The listing builds one solid part. Answer for the finished solid, in the listing's coordinates (mm). A direction names the side the tool comes from. Give positions to 0.01 mm unless a question says otherwise; leave off trailing zeros. Loops run counter-clockwise (first coordinate to the right, second up) from the corner with the lowest first, then second, coordinate; pieces in that order, holes last.
Item 1: Section B-B, the plane y = 0 is taken. Give the vertices of the cut face in (x, z).
Item 2: A tool of negligible diameter and unlimited length cuts with its end or side. For faces 1 (the face through (-5, -1, 8)), 2 (the face through (-2.1, 1.3, 6.7)), 3 (the face through (-1.287, 0.103, 5.179)), 4 (the face through (-5, 1, 8)), 5 (the face through (-7, 0, 9.7)), from which of +Z, -Z, +X, -X, +Y, -Y can it reach the whole face along a straight path? Write none if from no direction.
Item 3: Consider line 1 along X through (y, z) = (0, 6); line 2 along Z through (x, y) = (-2.25, 1.5); line 3 along X through (y, z) = (0, 7.5). Determine where each line is inside the solid, lowest interval first.
Item 4: Section A-A, the plane z = 6.25 is taken. Give the vertices of the cut face in (x, y), and give its area (3 significant figures).
Item 5: Section C-C, the plane x = 1.5 is taken. Give the vertices of the cut face in (y, z).
Item 6: Section D-D, the plane z = 7.25 is taken. Give the vertices of the cut face in (x, y), and give its area (3 significant figures).
Item 7: The mould has two halves that part along Y. Classify faces 6 (the face through (-6.171, 2.177, 4.317)), 7 (the face through (-4, 0, 2)), 8 (the face through (1, -2, 3.5)): pulls with the +Y half, pulls with the -Y half, needs draft (parallel to the pull), parting line crosses it, or undercut.
Item 8: Each of these flat-tipped pins is pushed along its axis until it touches: pin 1 Ø1.4 at (x, y) = (0, -0.5) entering from +Z; pin 2 Ø4 at (y, z) = (2, 7) entering from -X; pin 3 Ø2.5 at (x, y) = (1.06, 0) entering from +Z; pin 4 Ø1.5 at (x, z) = (-4, 8) entering from -Y. Where does it stop, or does it pass through?
from build123d import *
from build123d.topology import SkipClean

# Parameters (mm, degrees)
SKETCH1_R           = 2.35
BOSS_EXTRUDE1_DEPTH = 6.7
BOSS_EXTRUDE2_DEPTH = 3
CUT_EXTRUDE1_DEPTH  = 2
SKETCH4_R           = 2.35
SKETCH4_R_2         = 1.45
BOSS_EXTRUDE3_DEPTH = 1.5


with BuildPart() as part:
    # Sketch1 → Boss-Extrude1 (new body)
    with BuildSketch(Plane.XY):
        with BuildLine():
            Line((-1.533260445, 2.35), (-10.939517975, 2))
            ThreePointArc((-10.939517975, 2), (-12.939517975, 0), (-10.939517975, -2))
            Line((-10.939517975, -2), (-1.533260445, -2.35))
            ThreePointArc((-1.533260445, -2.35), (4.560482025, 0), (-1.533260445, 2.35))
        make_face()
        with Locations((1.060482025, 0)):
            Circle(SKETCH1_R, mode=Mode.SUBTRACT)
    extrude(amount=BOSS_EXTRUDE1_DEPTH)

    # Sketch2 → Boss-Extrude2 (add)
    with SkipClean():  # the faces are left unmerged after this step: merging them gives an invalid solid
        with BuildSketch(Plane.XY.offset(6.7)):
            with BuildLine():
                Line((-8.939517975, 1), (-1.289517975, 1))
                ThreePointArc((-1.289517975, 1), (-1.18252076, 0.99425932), (-1.076752018, 0.977103192))
                ThreePointArc((-1.076752018, 0.977103192), (-1.289517975, 0), (-1.076752018, -0.977103192))
                ThreePointArc((-1.076752018, -0.977103192), (-1.18252076, -0.99425932), (-1.289517975, -1))
                Line((-1.289517975, -1), (-8.939517975, -1))
                ThreePointArc((-8.939517975, -1), (-9.065522268, -0.992029696), (-9.189517975, -0.968245837))
                ThreePointArc((-9.189517975, -0.968245837), (-12.939517975, 0), (-9.189517975, 0.968245837))
                ThreePointArc((-9.189517975, 0.968245837), (-9.065522268, 0.992029696), (-8.939517975, 1))
            make_face()
        extrude(amount=BOSS_EXTRUDE2_DEPTH)

    # Sketch3 → Cut-Extrude1 (cut)
    with SkipClean():  # the faces are left unmerged after this step: merging them gives an invalid solid
        with BuildSketch(Plane(origin=(0, 0, 0), x_dir=(-1, 0, 0), z_dir=(0, 0, -1))):
            with BuildLine():
                Line((10.939517975, 2), (1.533260445, 2.35))
                ThreePointArc((1.533260445, 2.35), (-4.560482025, 0), (1.533260445, -2.35))
                Line((1.533260445, -2.35), (10.939517975, -2))
                ThreePointArc((10.939517975, -2), (12.939517975, 0), (10.939517975, 2))
            make_face()
        extrude(amount=-CUT_EXTRUDE1_DEPTH, mode=Mode.SUBTRACT)

    # Sketch4 → Boss-Extrude3 (add)
    with SkipClean():  # the faces are left unmerged after this step: merging them gives an invalid solid
        with BuildSketch(Plane(origin=(0, 0, 2), x_dir=(-1, 0, 0), z_dir=(0, 0, -1))):
            with Locations((-1.060482025, 0)):
                Circle(SKETCH4_R)
            with Locations((-1.060482025, 0)):
                Circle(SKETCH4_R_2, mode=Mode.SUBTRACT)
        extrude(amount=-BOSS_EXTRUDE3_DEPTH)


solid = part.part
Worked answers:
1. outline: (-12.94, 2) - (-0.39, 2) - (-0.39, 3.5) - (-1.29, 3.5) - (-1.29, 9.7) - (-12.94, 9.7) - close; (2.51, 2) - (4.56, 2) - (4.56, 6.7) - (3.41, 6.7) - (3.41, 3.5) - (2.51, 3.5) - close
2. face 1: +Z, +X, -Y
2. face 2: +Z, +X
2. face 3: +Z
2. face 4: +Z, +X, +Y
2. face 5: +Z, +X, -X, +Y, -Y
3. line 1: x = -12.94 to -1.29, 3.41 to 4.56
3. line 2: z = 2 to 6.7
3. line 3: x = -12.94 to -1.29
4. outline: (-10.94, -2) - (-1.53, -2.35) arc R3.5 ccw (long way) to (-1.53, 2.35) - (-10.94, 2) arc R2 ccw to start; hole circle Ø4.7 at (1.06, 0)
4. area: 65.4 mm2
5. outline: (-3.47, 2) - (-1.38, 2) - (-1.38, 3.5) - (-2.31, 3.5) - (-2.31, 6.7) - (-3.47, 6.7) - close; (1.38, 2) - (3.47, 2) - (3.47, 6.7) - (2.31, 6.7) - (2.31, 3.5) - (1.38, 3.5) - close
6. outline: (-9.19, -0.97) arc R1 ccw to (-8.94, -1) - (-1.29, -1) arc R1 ccw to (-1.08, -0.98) arc R2.35 cw to (-1.08, 0.98) arc R1 ccw to (-1.29, 1) - (-8.94, 1) arc R1 ccw to (-9.19, 0.97) arc R2 ccw (long way) to start
6. area: 28.2 mm2
7. face 6: pulls with the +Y half
7. face 7: needs draft
7. face 8: undercut
8. pin 1: stops at z = 3.5
8. pin 2: stops at x = -12.94
8. pin 3: passes through
8. pin 4: stops at y = -1
